The figure shows three views and two pictorial views of one solid part (mm, origin at its lowest corner). Answer the questions. Coordinates: 2 decimals unless noted, no trailing zeros. Order: outer loops, then holes, each group sorted by start corner. A loop starts at its lowest first (then second) coordinate and runs counter-clockwise, first axis right, second up. Notation, with made-up numbers: (27, -25) - (82, -25) arc R29 ccw to (82, -5) - close; hole circle Ø1 at (11, 77). An arc over 180 degrees is marked (long way). Use one line per item in the form item = value. Start each with the question number.
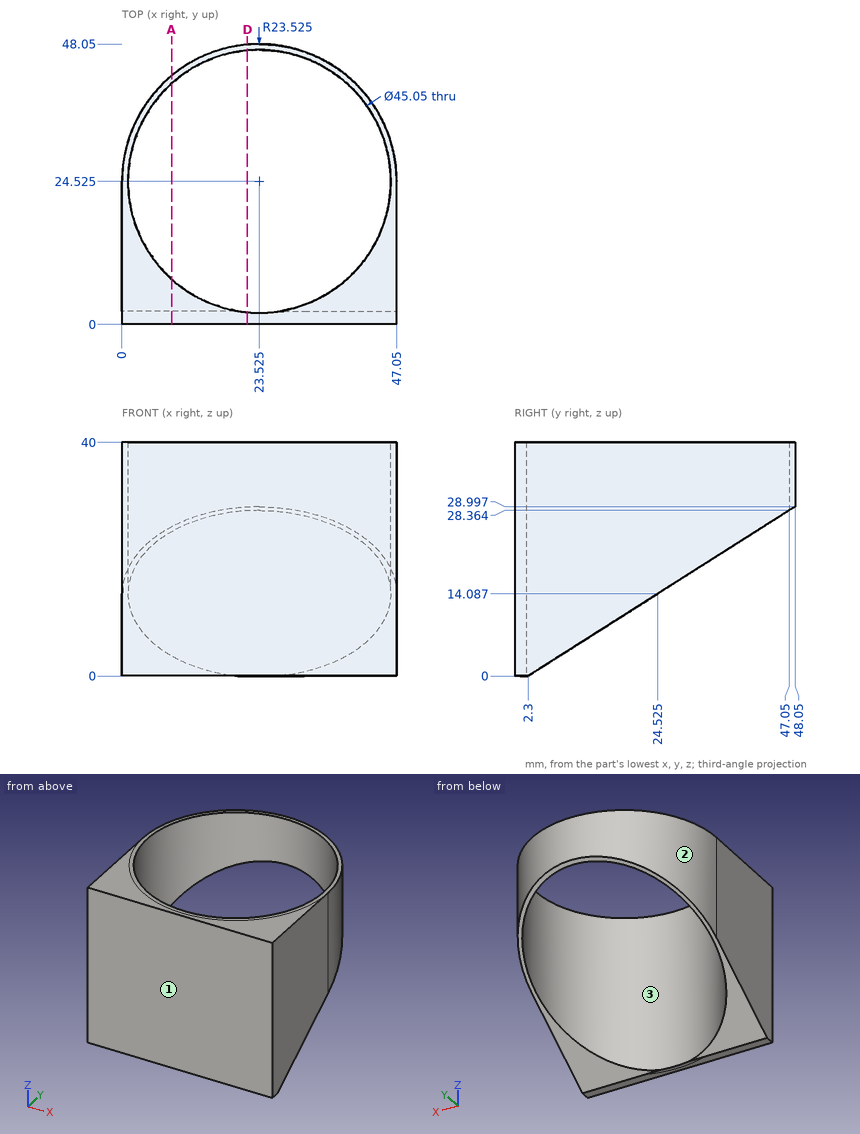
Q1. For a pull along X with two mould halves and no side action, classify the marked faces 1, 2 and 3 as +X half, -X half, draft (parallel to the pull), parting line (faces both ways), or undercut.
Q2. Consider probe 1 along Y at (x, z) = (23, 32) (1 decimal); probe 2 along X at (y, z) = (19.5, 25.5); probe 3 along Y at (x, z) = (29, 36) (1 decimal). Determine where each line is inside the solid, lowest interval first.
Q3. A cutting plane is placed at D-D (x = 21.5). Give the vertices of the cut face in (y, z) (1 decimal).
Q4. Given P1, Ø1.5, axis at x = 28.5, z = 24.5, coming from the +Y side; P2, Ø3, axis at y = 27.5, z = 14, coming from the -X side, each flat-ended and moving along its own axis, determine where each tip first touches the part or whether it passes through.
Q5. A cutting plane is placed at A-A (x = 8.5). Give the vertices of the cut face in (y, z).
Result sheet:
q1.face_1 = draft
q1.face_2 = parting line
q1.face_3 = undercut
q2.probe_1 = 0 to 2, 47 to 48
q2.probe_2 = 0 to 1.57, 45.48 to 47.05
q2.probe_3 = 0 to 2.7, 46.4 to 47.4
q3.outline = (0, 0) - (2.1, 0) - (2.1, 40) - (0, 40) - close; (47, 28.3) - (48, 28.9) - (48, 40) - (47, 40) - close
q4.P1 = 2.74
q4.P2 = through
q5.outline = (0, 0) - (2.3, 0) - (7.74, 3.45) - (7.74, 40) - (0, 40) - close; (41.31, 24.72) - (42.63, 25.56) - (42.63, 40) - (41.31, 40) - close
